Here's how the part is built. I have some questions about the finished solid (model axes, mm). Round coordinates to 2 decimals unless told otherwise and drop trailing zeros. Write each loop counter-clockwise with the first axis right and the second up, starting at its lowest first coordinate (ties: lowest second). Pieces come first, ordered by that corner, then holes. Notation, with made-up numbers: (-13, 49) -> (40, 49) arc R17 ccw to (40, 75) -> close; hole circle Ø9 at (79.25, 54.25). An arc over 180 degrees is marked (long way). Answer as CSV lines item,"result".
```python
from build123d import *

# Parameters (mm, degrees)
F0_W     = 25
F0_H     = 25
F1_DEPTH = 7.5
F2_R     = 1.35
F2_R_2   = 1.4
F2_R_3   = 1.45
F2_R_4   = 1.5
F2_R_5   = 1.55
F2_R_6   = 1.6
F2_R_7   = 1.65
F3_DEPTH = 7.501
F4_R     = 5


with BuildPart() as f1:
    # F0 (on Top) → F1 (new body)
    with BuildSketch(Plane.XY):
        Rectangle(F0_W, F0_H)
    extrude(amount=F1_DEPTH)

    # F2 (on face) → F3 (cut, through all)
    with BuildSketch(Plane.XY.offset(7.5)):
        with Locations((-6.25, 9.375)):
            Circle(F2_R)
        with Locations((-6.25, 3.125)):
            Circle(F2_R_2)
        with Locations((-6.25, -3.125)):
            Circle(F2_R_3)
        with Locations((-6.25, -9.375)):
            Circle(F2_R_4)
        with Locations((6.25, 9.375)):
            Circle(F2_R_5)
        with Locations((6.25, 3.125)):
            Circle(F2_R_6)
        with Locations((6.25, -3.125)):
            Circle(F2_R_7)
    extrude(amount=-F3_DEPTH, mode=Mode.SUBTRACT)

    # F4
    f4_edges = [f1.edges().sort_by_distance(p)[0] for p in [
        (-12.5, 12.5, 3.75),
        (-12.5, -12.5, 3.75),
        (12.5, -12.5, 3.75),
        (12.5, 12.5, 3.75),
    ]]
    fillet(f4_edges, radius=F4_R)


solid = f1.part
```
1. If we mould it in two halves opening along X, with no side actions, what happens to faces 1 (the face through (-7.7, -3.1, 3.8)), 2 (the face through (0, -12.5, 4)), 3 (the face through (-11.07, -11, 3.8))? For each: released by +X, released by -X, zero draft, split by the parting line, or undercut.
Numbers:
face 1,"undercut"
face 2,"zero draft"
face 3,"released by -X"
2. Suppose I cut it at B-B on x = -6.25. Please give me the cut outline in (y, z) (3 decimals), and give its area (3 significant figures).
Numbers:
outline,"(-12.5, 0) -> (-10.875, 0) -> (-10.875, 7.5) -> (-12.5, 7.5) -> close; (-7.875, 0) -> (-4.575, 0) -> (-4.575, 7.5) -> (-7.875, 7.5) -> close; (-1.675, 0) -> (1.725, 0) -> (1.725, 7.5) -> (-1.675, 7.5) -> close; (4.525, 0) -> (8.025, 0) -> (8.025, 7.5) -> (4.525, 7.5) -> close; (10.725, 0) -> (12.5, 0) -> (12.5, 7.5) -> (10.725, 7.5) -> close"
area,"102 mm^2"
3. Suppose I cut it at D-D on y = -8.25. Please give me the cut outline in (x, z), and give its area (3 significant figures).
Numbers:
outline,"(-12.44, 0) -> (-7.24, 0) -> (-7.24, 7.5) -> (-12.44, 7.5) -> close; (-5.26, 0) -> (12.44, 0) -> (12.44, 7.5) -> (-5.26, 7.5) -> close"
area,"172 mm^2"
4. Suppose I cut it at A-A on x = 6.25. Please give me the cut outline in (y, z) (3 decimals), and give its area (4 significant figures).
Numbers:
outline,"(-12.5, 0) -> (-4.775, 0) -> (-4.775, 7.5) -> (-12.5, 7.5) -> close; (-1.475, 0) -> (1.525, 0) -> (1.525, 7.5) -> (-1.475, 7.5) -> close; (4.725, 0) -> (7.825, 0) -> (7.825, 7.5) -> (4.725, 7.5) -> close; (10.925, 0) -> (12.5, 0) -> (12.5, 7.5) -> (10.925, 7.5) -> close"
area,"115.5 mm^2"
5. Suppose I cut it at C-C on y = -4.25. Please give me the cut outline in (x, z), and give its area (3 significant figures).
Numbers:
outline,"(-12.5, 0) -> (-7.16, 0) -> (-7.16, 7.5) -> (-12.5, 7.5) -> close; (-5.34, 0) -> (5.04, 0) -> (5.04, 7.5) -> (-5.34, 7.5) -> close; (7.46, 0) -> (12.5, 0) -> (12.5, 7.5) -> (7.46, 7.5) -> close"
area,"156 mm^2"
6. If I drill on line 1 (X direction, y = -3.5, z = 3); line 2 (Y direction, x = -6.25, z = 2.25) (3 decimals); line 3 (Y direction, x = 6.25, z = 2.25) (3 decimals), over which ranges is the centre line in solid material (lowest first)?
Numbers:
line 1,"x = -12.5 to -7.65, -4.85 to 4.64, 7.86 to 12.5"
line 2,"y = -12.5 to -10.875, -7.875 to -4.575, -1.675 to 1.725, 4.525 to 8.025, 10.725 to 12.5"
line 3,"y = -12.5 to -4.775, -1.475 to 1.525, 4.725 to 7.825, 10.925 to 12.5"
